Can you work these out from the model? Positions are in its coordinate system, mm. Face numbers are marked on the shaded views. A direction names the side the tool comes from. Round coordinates to 2 decimals unless told otherwise and drop trailing zeros. Loops run counter-clockwise (first coordinate to the right, second up) from the corner with the lowest first, then second, coordinate; pieces in that order, holes last. Notation, with made-up numbers: (10.25, -35) -> (63.25, -35) arc R18 cw to (63.25, -5) -> close; hole circle Ø4 at (-16, 19.5). An arc over 180 degrees is marked (long way). Write item = value, one per line.
from build123d import *

# Parameters (mm, degrees)
BOSS_EXTRUDE1_DEPTH                                 = 6.35
SKETCH2_W                                           = 12.7
SKETCH2_H                                           = 12.7
BOSS_EXTRUDE2_DEPTH                                 = 10.16
CBORE_FOR_6_BINDING_HEAD_MACHINE_SCREW1_D           = 3.7973
CBORE_FOR_6_BINDING_HEAD_MACHINE_SCREW1_CBORE_D     = 7.9375
CBORE_FOR_6_BINDING_HEAD_MACHINE_SCREW1_CBORE_DEPTH = 4.7498


with BuildPart() as part:
    # Sketch1 → Boss-Extrude1 (new, symmetric)
    with BuildSketch(Plane.XY):
        with BuildLine():
            Line((-3.175, 4.7625), (-3.175, 6.35))
            Line((-3.175, 6.35), (3.175, 6.35))
            Line((3.175, 6.35), (3.175, -6.35))
            Line((3.175, -6.35), (-3.175, -6.35))
            Line((-3.175, -6.35), (-3.175, -4.7625))
            ThreePointArc((-3.175, -4.7625), (1.5875, 0), (-3.175, 4.7625))
        make_face()
    extrude(amount=BOSS_EXTRUDE1_DEPTH, both=True)

    # Sketch2 → Boss-Extrude2 (add)
    with BuildSketch(Plane.XY.offset(6.35)):
        with Locations((-3.175, 0)):
            Rectangle(SKETCH2_W, SKETCH2_H)
    extrude(amount=BOSS_EXTRUDE2_DEPTH)

    # CBORE for #6 Binding Head Machine Screw1 (through all)
    with Locations(Plane(origin=(3.175, 0, 0), x_dir=(0, 0, -1), z_dir=(1, 0, 0))):
        with Locations((-11.43, 0)):
            CounterBoreHole(CBORE_FOR_6_BINDING_HEAD_MACHINE_SCREW1_D / 2, CBORE_FOR_6_BINDING_HEAD_MACHINE_SCREW1_CBORE_D / 2, CBORE_FOR_6_BINDING_HEAD_MACHINE_SCREW1_CBORE_DEPTH)


solid = part.part
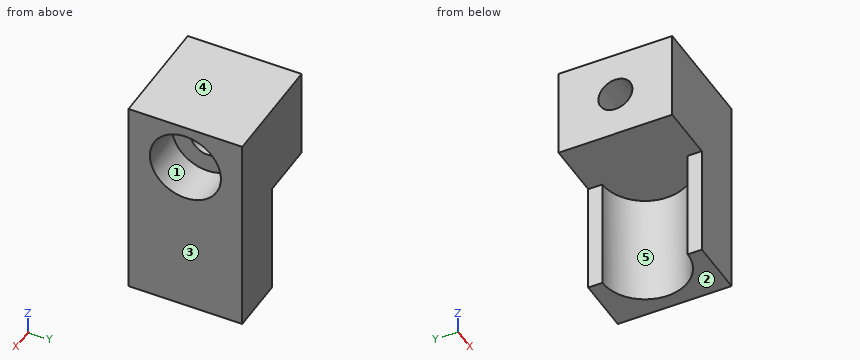
1. I need wall thicknesses on line 1 (Y direction, x = -1, z = 11.5); line 2 (Y direction, x = -3, z = 11.43); line 3 (Z direction, x = -4.25, y = 3.75). Which ranges of each line are inside material? Lowest first, please. Write a range as [from, to].
Entries:
line_1 = [-6.35, -3.97], [3.97, 6.35]
line_2 = [-6.35, -1.9], [1.9, 6.35]
line_3 = [6.35, 16.51]
2. Suppose I cut it at C-C, the plane x = 0.25. List the corners of the cut face in (y, z) for me, and give its area (3 significant figures).
Entries:
outline = (-6.35, -6.35) -> (-3.31, -6.35) -> (-3.31, 6.35) -> (3.31, 6.35) -> (3.31, -6.35) -> (6.35, -6.35) -> (6.35, 16.51) -> (-6.35, 16.51) -> close; hole circle Ø7.94 at (0, 11.43)
area = 157 mm²
3. I'm going to push flat-ended pins straight in: pin 1 (4 mm diameter, centred on y = -0.5, z = 10, fed in from +X); pin 2 (2 mm diameter, centred on x = -4, z = -3, fed in from -Y); pin 3 (1.3 mm diameter, centred on y = 6, z = -3, fed in from -X) (3 decimals); pin 4 (1 mm diameter, centred on x = -8, y = 4.5, fed in from -Z). Where does each tip first touch, or does it pass through?
Entries:
pin_1 = -1.57
pin_2 = -6.35
pin_3 = -3.175
pin_4 = 6.35
4. For the marked faces 4 and 5, which set-ups out of +Z, -Z, +X, -X, +Y, -Y let a thin tool reach every point of the face, with its end or its side?
Entries:
face_4 = +Z, +X, -X, +Y, -Y
face_5 = -Z, -X
5. We'd pull the mould along Z, two halves only. Please class the marked faces 1, 2 and 3: released by +Z, released by -Z, zero draft, split by the parting line, or undercut.
Entries:
face_1 = undercut
face_2 = released by -Z
face_3 = zero draft
6. Suppose I cut it at A-A, the plane z = 11.43. List the corners of the cut face in (x, y) for me (3 decimals), and give its area (3 significant figures).
Entries:
outline = (-9.525, -6.35) -> (3.175, -6.35) -> (3.175, -3.969) -> (-1.575, -3.969) -> (-1.575, -1.899) -> (-9.525, -1.899) -> close; (-9.525, 1.899) -> (-1.575, 1.899) -> (-1.575, 3.969) -> (3.175, 3.969) -> (3.175, 6.35) -> (-9.525, 6.35) -> close
area = 93.4 mm²
